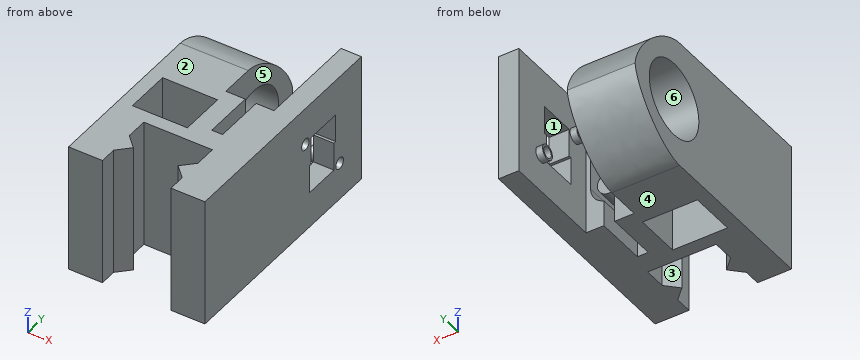
```python
from build123d import *

# Parameters (mm, degrees)
SKETCH1_W                = 16.2
SKETCH1_H                = 13.5
BOSS_EXTRUDE1_DEPTH      = 19
SKETCH2_W                = 20
SKETCH2_H                = 38
BOSS_EXTRUDE2_DEPTH      = 30
FILLET2_SIZE             = 20
SKETCH7_W                = 6
SKETCH7_H                = 38
BOSS_EXTRUDE6_DEPTH      = 30
CUT_EXTRUDE1_DEPTH       = 69.038885968
CUT_EXTRUDE1_DEPTH_BACK  = 31
SKETCH3_R                = 11.075
SKETCH5_W                = 2.5
SKETCH5_H                = 38
BOSS_EXTRUDE3_DEPTH      = 30
SKETCH11_R               = 3.5
CUT_EXTRUDE5_DEPTH       = 15
SKETCH9_R                = 2.2
BOSS_EXTRUDE7_DEPTH      = 8
M3_CLEARANCE_HOLE3_D     = 3.4
M3_CLEARANCE_HOLE3_DEPTH = 8
CUT_EXTRUDE6_DEPTH       = 10


with BuildPart() as part:
    # Sketch1 → Boss-Extrude1 (new, symmetric)
    with BuildSketch(Plane.XY):
        Polygon((-10.1, 0), (10.1, 0), (10.1, -6.5), (6.6, -10), (10.1, -13.5), (10.1, -18.5), (20.1, -18.5), (20.1, 21.5), (-20.1, 21.5), (-20.1, -18.5), (-10.1, -18.5), (-10.1, -13.5), (-6.6, -10), (-10.1, -6.5), align=None)
        with Locations((-8, 10.75)):
            Rectangle(SKETCH1_W, SKETCH1_H, mode=Mode.SUBTRACT)
    extrude(amount=BOSS_EXTRUDE1_DEPTH, both=True)

    # Sketch2 → Boss-Extrude2 (add)
    with BuildSketch(Plane(origin=(0, 21.5, 0), x_dir=(1, 0, 0), z_dir=(0, 1, 0))):
        with Locations((-10.1, 0)):
            Rectangle(SKETCH2_W, SKETCH2_H)
    extrude(amount=BOSS_EXTRUDE2_DEPTH)

    # Fillet2
    # a fillet whose section is not a circle: 20 mm, written as the material it takes off along each edge
    with BuildSketch(Plane(origin=(-70.1, 51.5, -19), x_dir=(0, 0, 1), z_dir=(1, 0, 0)), Plane(origin=(49.9, 51.5, 19), x_dir=(0, 0, -1), z_dir=(-1, 0, 0))) as fillet2_piece_1:
        with BuildLine():
            Bezier((FILLET2_SIZE, 0), (0, 0), (0, FILLET2_SIZE), weights=[1, 0.428571429, 1])
            Line((0, FILLET2_SIZE), (0, 0))
            Line((0, 0), (FILLET2_SIZE, 0))
        make_face()
    extrude(amount=120, mode=Mode.SUBTRACT)

    # Sketch7 → Boss-Extrude6 (add)
    with BuildSketch(Plane(origin=(0, 21.5, 0), x_dir=(1, 0, 0), z_dir=(0, 1, 0))):
        with Locations((17.1, 0)):
            Rectangle(SKETCH7_W, SKETCH7_H)
    extrude(amount=BOSS_EXTRUDE6_DEPTH)

    # Sketch3 → Cut-Extrude1 (cut, two sides: drawn at the far end of the back side and taken through both)
    with BuildSketch(Plane.ZY.offset(20.1).offset(-CUT_EXTRUDE1_DEPTH_BACK)):
        with Locations(Location((0, 34, 0), (0, 0, 90))):
            Circle(SKETCH3_R)
    extrude(amount=CUT_EXTRUDE1_DEPTH + CUT_EXTRUDE1_DEPTH_BACK, mode=Mode.SUBTRACT)

    # Sketch5 → Boss-Extrude3 (add)
    with BuildSketch(Plane(origin=(0, 21.5, 0), x_dir=(1, 0, 0), z_dir=(0, 1, 0))):
        with Locations((18.85, 0)):
            Rectangle(SKETCH5_W, SKETCH5_H)
    extrude(amount=BOSS_EXTRUDE3_DEPTH)

    # Sketch11 → Cut-Extrude5 (cut)
    with BuildSketch(Plane(origin=(0, 21.5, 0), x_dir=(1, 0, 0), z_dir=(0, 1, 0))):
        with BuildLine():
            Line((5.63, -11.262128847), (5.63, -19))
            Line((5.63, -19), (8.83, -19))
            Line((8.83, -19), (8.83, -11.262128847))
            ThreePointArc((8.83, -11.262128847), (11.648710219, -9.274904579), (12.73, -6))
            Line((12.73, -6), (12.73, 6))
            ThreePointArc((12.73, 6), (11.648710219, 9.274904579), (8.83, 11.262128847))
            Line((8.83, 11.262128847), (8.83, 19))
            Line((8.83, 19), (5.63, 19))
            Line((5.63, 19), (5.63, 11.262128847))
            ThreePointArc((5.63, 11.262128847), (2.811289781, 9.274904579), (1.73, 6))
            Line((1.73, 6), (1.73, -6))
            ThreePointArc((1.73, -6), (2.811289781, -9.274904579), (5.63, -11.262128847))
        make_face()
        with Locations(Location((7.23, 6, 0), (0, 0, 180))):
            Circle(SKETCH11_R, mode=Mode.SUBTRACT)
        with Locations(Location((7.23, -6, 0), (0, 0, 180))):
            Circle(SKETCH11_R, mode=Mode.SUBTRACT)
    extrude(amount=-CUT_EXTRUDE5_DEPTH, mode=Mode.SUBTRACT)

    # Sketch9 → Boss-Extrude7 (add)
    with BuildSketch(Plane(origin=(20.1, 0, 0), x_dir=(0, 0, -1), z_dir=(1, 0, 0))):
        with Locations(Location((7.85, 41.75, 0), (0, 0, 90))):
            Circle(SKETCH9_R)
        with Locations(Location((-7.85, 26.45, 0), (0, 0, 90))):
            Circle(SKETCH9_R)
    extrude(amount=-BOSS_EXTRUDE7_DEPTH)

    # M3 Clearance Hole3
    with Locations(Plane(origin=(12.1, 41.75, -7.85), x_dir=(0, -1, 0), z_dir=(-1, 0, 0))):
        with Locations((0, 0), (15.3, 15.7)):
            Hole(M3_CLEARANCE_HOLE3_D / 2, depth=M3_CLEARANCE_HOLE3_DEPTH)

    # Sketch19 → Cut-Extrude6 (cut)
    with BuildSketch(Plane(origin=(20.1, 0, 0), x_dir=(0, 0, -1), z_dir=(1, 0, 0))):
        Polygon((0, 39.2), (8.35, 39.2), (8.35, 28.2), (0, 28.2), (0, 29), (-8.35, 29), (-8.35, 40), (0, 40), align=None)
    extrude(amount=-CUT_EXTRUDE6_DEPTH, mode=Mode.SUBTRACT)


solid = part.part
```
Could you check a few things on this model? Use its own coordinates, in mm. Face numbers are marked on the shaded views. A direction names the side the tool comes from. Give positions to 0.01 mm unless a question says otherwise; leave off trailing zeros. Loops run counter-clockwise (first coordinate to the right, second up) from the corner with the lowest first, then second, coordinate; pieces in that order, holes last. Notation, with made-up numbers: (-32.75, 85.5) -> (8.25, 85.5) arc R14 ccw to (8.25, 108.5) -> close; hole circle Ø3 at (33, -29.5). An arc over 180 degrees is marked (long way). Put each result on its own line as item: value.
(1) I'm going to push flat-ended pins straight in: pin 1 Ø5.5 at (x, z) = (7, -7) entering from +Y; pin 2 Ø8 at (x, z) = (-5.5, 8) entering from +Y; pin 3 Ø1 at (y, z) = (44.5, 15) entering from -X. Where does each tip first touch, or does it pass through?
Computed:
pin 1: y = 21.5
pin 2: y = 50.23
pin 3: x = 14.1
(2) Please list where these lines run through material, in increasing order: probe 1 along X at (y, z) = (17, 13); probe 2 along X at (y, z) = (-1, 16.5); probe 3 along X at (y, z) = (30, -11.5). Write a range as [from, to].
Computed:
probe 1: [-20.1, -16.1], [0.1, 5.63], [8.83, 20.1]
probe 2: [-20.1, -10.1], [10.1, 20.1]
probe 3: [-20.1, -0.1], [14.1, 20.1]
(3) Imagine slicing it at A-A on y = 14. Write out the boundary of the cut face in (x, z), plus the area to 3 significant figures.
Computed:
outline: (-20.1, -19) -> (-16.1, -19) -> (-16.1, 19) -> (-20.1, 19) -> close; (0.1, -19) -> (5.63, -19) -> (5.63, -11.26) arc R5.5 cw to (1.73, -6) -> (1.73, 6) arc R5.5 cw to (5.63, 11.26) -> (5.63, 19) -> (0.1, 19) -> close; circle Ø7 at (7.23, -6); circle Ø7 at (7.23, 6); (8.83, -19) -> (20.1, -19) -> (20.1, 19) -> (8.83, 19) -> (8.83, 11.26) arc R5.5 cw to (12.73, 6) -> (12.73, -6) arc R5.5 cw to (8.83, -11.26) -> close
area: 713 mm^2
(4) For the marked faces 1, 2 and 3, which set-ups out of +Z, -Z, +X, -X, +Y, -Y let a thin tool reach every point of the face, with its end or its side?
Computed:
face 1: +X, -X
face 2: +Z, +X, -X, +Y, -Y
face 3: +Z, -Z
(5) Thinking about a two-plate mould opening in Z: for the marked faces 4, 5 and 6, which applies, pulls with the +Z half, pulls with the -Z half, needs draft (parallel to the pull), parting line crosses it, or undercut?
Computed:
face 4: pulls with the -Z half
face 5: needs draft
face 6: undercut
(6) Imagine slicing it at B-B on x = -1. State how many separate pieces and enclosed holes the cut face has, plus the area to 3 significant figures.
Computed:
separate pieces: 2
enclosed holes: 1
area: 831 mm^2
